```python
from build123d import *

# Parameters (mm, degrees)
F0_W        = 74.5595730841
F0_H        = 68.4390123934
F1_DEPTH    = 127
F2_T        = -2.54
F3_T1_DEPTH = 451.5844547388
F3_T3_DEPTH = 451.5844547388
F6_W        = 45.6260088831
F6_H        = 7.7898120508
F7_DEPTH    = 76.2
F8_R        = 24.5284097937
F11_W       = 38.0337639379
F11_H       = 74.3822181045
F12_DEPTH   = 5.08


# Not quite as in the source:
# - a fillet or chamfer that OpenCascade refuses, or shapes differently, is made with other operations: its cross-section is extruded or revolved along the edge and cut away or added
# - the program builds the solid bodies; features that only make, move or delete a surface that nothing else refers to are left out


with BuildPart() as f1:
    # F0 (on Top) → F1 (new body)
    with BuildSketch(Plane.XY):
        with Locations((2.225657925, 3.8948999718)):
            Rectangle(F0_W, F0_H)
    extrude(amount=F1_DEPTH)

    # F2
    f2_openings = [f1.faces().sort_by_distance(p)[0] for p in [
        (2.225658, 3.8949, 127),
        (39.505444, 3.8949, 63.5),
    ]]
    offset(amount=F2_T, openings=f2_openings)

    # F3: fillet of radius 91.3683264816 on 2 edges, made by hand

    # F3_s2 → F3_t1 (cut)
    with BuildSketch(Plane.XZ.offset(-196.7376211445)):
        with BuildLine():
            ThreePointArc((-35.054128617, 127), (18.4363311824, 95.5536973082), (39.5054444671, 37.1911090522))
            Line((39.5054444671, 37.1911090522), (39.5054444671, 127))
            Line((39.5054444671, 127), (-35.054128617, 127))
        make_face()
    extrude(amount=F3_T1_DEPTH, mode=Mode.SUBTRACT)

    # F3_s4 → F3_t3 (cut)
    with BuildSketch(Plane.XZ.offset(-262.6366335379)):
        with BuildLine():
            ThreePointArc((-35.054128617, 127), (18.4363311824, 95.5536973082), (39.5054444671, 37.1911090522))
            Line((39.5054444671, 37.1911090522), (39.5054444671, 127))
            Line((39.5054444671, 127), (-35.054128617, 127))
        make_face()
    extrude(amount=F3_T3_DEPTH, mode=Mode.SUBTRACT)

    # F4: F1 across plane


with BuildPart() as f1_1:
    add(f1.part)
    add(f1.part.mirror(Plane.XZ))

    # F5: F1 across plane


with BuildPart() as f1_2:
    add(f1_1.part)
    add(f1_1.part.mirror(Plane.XY))

    # F6 (on face) → F7 (join)
    with BuildSketch(Plane(origin=(0, 0, -2.54), x_dir=(1, 0, 0), z_dir=(0, 0, -1))):
        with Locations((-9.5800887793, 0)):
            Rectangle(F6_W, F6_H)
    extrude(amount=F7_DEPTH)

    # F8
    f8_edges = [f1_2.edges().sort_by_distance(p)[0] for p in [
        (13.232916, 0, -78.74),
    ]]
    fillet(f8_edges, radius=F8_R)

    # F9: F1 across plane


with BuildPart() as f1_3:
    add(f1_2.part)
    add(f1_2.part.mirror(Plane.XY))

    # F10: F1 across face


with BuildPart() as f1_4:
    add(f1_3.part)
    add(f1_3.part.mirror(Plane(origin=(-35.054128617, 0, 0), x_dir=(0, -1, 0), z_dir=(-1, 0, 0))))

    # F11 (on face) → F12 (join)
    with BuildSketch(Plane(origin=(0, 38.1144061685, 0), x_dir=(-1, 0, 0), z_dir=(0, 1, 0))):
        with Locations((32.8460000455, 0)):
            Rectangle(F11_W, F11_H)
    extrude(amount=F12_DEPTH)


solid = f1_4.part
```
The model under review builds one solid part; all positions refer to its coordinate system, in mm. A direction names the side the tool comes from. Round coordinates to 2 decimals unless told otherwise and drop trailing zeros. Write each loop counter-clockwise with the first axis right and the second up, starting at its lowest first coordinate (ties: lowest second). Pieces come first, ordered by that corner, then holes. Notation, with made-up numbers: M 33,9 L 45,9 A24 cw 45,40 Z; hole C 10.5,8 d10. An arc over 180 degrees is marked long. Use CSV: the item, a comma, the result in double quotes. Start each with the question number.
(1) The part is to be moulded in two halves that separate along Y. For faces 6 (the face through (13.233, 0, 28)), 7 (the face through (-33, 41, -37.191)), say which applies: +Y half, -Y half, draft (parallel to the pull), parting line (faces both ways), or undercut.
(2) We need section C-C, the plane x = 16. State the section outline as (y, z) points.
(3) For line 1 along Y through (x, z) = (-79, -55); line 2 along Y through (x, z) = (-63.5, -83); line 3 along Y through (x, z) = (-16, 8.5), list the stretches that pass through material, from the lowest coordinate up.
(4) Clearance check with flat-ended pins moving along their axes: P1, Ø8, axis at x = -3, y = 12, coming from the +Z side; P2, Ø1, axis at y = 2.5, z = 61.5, coming from the +X side; P3, Ø2, axis at y = 31, z = 77, coming from the -X side. State where each tip first meets the part, or that it passes through.
(5) We need section B-B, the plane z = 5. State how many separate pieces and enclosed holes the cut face has, then the cut area to 3 significant figures.
(6) Tool access review of faces 1 (the face through (-73, -27.785, 50)), 2 (the face through (39.505, 0, 0)), 3 (the face through (3, 33, 2.54)), 4 (the face through (3, -27.785, -50)), 5 (the face through (-73, -33, -2.54)): name each direction out of +Z, -Z, +X, -X, +Y, -Y from which nothing blocks a thin tool from reaching the whole face with its end or side.
(7) We need section D-D, the plane z = -87.5. State the section outline as (x, y) points, then the cut area to 3 significant figures.
(8) We need section A-A, the plane y = -11.5. State the section outline as (x, z) points, then the cut area to 3 significant figures.
Findings:
1,face 6,"undercut"
1,face 7,"draft"
2,outline,"M -38.11,-98.37 L -35.57,-98.37 L -35.57,-2.54 L -30.32,-2.54 L -30.32,-98.37 L -27.78,-98.37 L -27.78,-2.54 L 27.78,-2.54 L 27.78,-98.37 L 30.32,-98.37 L 30.32,-2.54 L 35.57,-2.54 L 35.57,-98.37 L 38.11,-98.37 L 38.11,98.37 L 35.57,98.37 L 35.57,2.54 L 30.32,2.54 L 30.32,98.37 L 27.78,98.37 L 27.78,2.54 L -27.78,2.54 L -27.78,98.37 L -30.32,98.37 L -30.32,2.54 L -35.57,2.54 L -35.57,98.37 L -38.11,98.37 Z"
3,line 1,"-38.11 to -35.57, -30.32 to -27.78, -3.89 to 3.89, 27.78 to 30.32, 35.57 to 38.11"
3,line 2,"-38.11 to -35.57, -30.32 to -27.78, 27.78 to 30.32, 35.57 to 38.11"
3,line 3,"-38.11 to -35.57, -30.32 to -27.78, -3.89 to 3.89, 27.78 to 30.32, 35.57 to 43.19"
4,P1,"z = 2.54"
4,P2,"x = 12.27"
4,P3,"x = -100.84"
5,separate pieces,"3"
5,enclosed holes,"0"
5,area,"2,750 mm^2"
6,face 1,"+Z, -X"
6,face 2,"+Z, -Z, +X, +Y, -Y"
6,face 3,"+Z, +X"
6,face 4,"-Z, +X"
6,face 5,"-Z, -X"
7,outline,"M -94.52,-38.11 L 24.41,-38.11 L 24.41,-35.57 L -32.51,-35.57 L -32.51,-30.32 L 24.41,-30.32 L 24.41,-27.78 L -32.51,-27.78 L -32.51,27.78 L 24.41,27.78 L 24.41,30.32 L -32.51,30.32 L -32.51,35.57 L 24.41,35.57 L 24.41,38.11 L -94.52,38.11 L -94.52,35.57 L -37.59,35.57 L -37.59,30.32 L -94.52,30.32 L -94.52,27.78 L -37.59,27.78 L -37.59,-27.78 L -94.52,-27.78 L -94.52,-30.32 L -37.59,-30.32 L -37.59,-35.57 L -94.52,-35.57 Z"
7,area,"1,540 mm^2"
8,outline,"M -109.61,-2.54 L -37.59,-2.54 L -37.59,-126.49 A91.37 ccw -35.05,-127 A91.37 ccw -32.51,-126.49 L -32.51,-2.54 L 39.51,-2.54 L 39.51,2.54 L -32.51,2.54 L -32.51,126.49 A91.37 ccw -35.05,127 A91.37 ccw -37.59,126.49 L -37.59,2.54 L -109.61,2.54 Z"
8,area,"2,020 mm^2"
